Autodesk Inventor part; units mm, degrees
sketch "Esboço1" plane through (0, 0, 0) normal (0, 1, 0) x (-1, 0, 0)
  line L0 (-50, 50) -> (50, 50)
  line L1 (50, 50) -> (50, -50)
  line L2 (50, -50) -> (-50, -50)
  line L3 (-50, -50) -> (-50, 50)
  line L4 (-50, 50) -> (50, -50) construction
  line L5 (50, 50) -> (-50, -50) construction
  line L6 (-40, 40) -> (40, 40)
  line L7 (40, 40) -> (40, -40)
  line L8 (40, -40) -> (-40, -40)
  line L9 (-40, -40) -> (-40, 40)
  line L10 (-40, 40) -> (40, -40) construction
  line L11 (40, 40) -> (-40, -40) construction
  point P0 (0, 0)
  dimension "d0" = 100
  dimension "d1" = 10
extrude "Extrusão1" add sketch "Esboço1" along normal mid plane 740
equation "\"Raio_vergadura\" = Espessura"
equation "\"Largura_alívio_de_vergadura\" = Espessura"
equation "\"Profundidade_alívio_de_vergadura\" = 0.5 * Espessura"
equation "\"Tamanho_alívio_de_dobra\" = 4 * Espessura"
equation "\"Remanescente_mínimo\" = 2 * Espessura"
equation "\"Raiodetransição\" = Raio_vergadura"
equation "\"Tamanho_de_raio_de_Jacobi\" = Raio_vergadura"
equation "\"TamanhoFolga\" = Espessura"
properties part number "Perna para Exercício"
Build history of the part. All positions in model axes, mm. A direction names the side the tool comes from. Coordinates: 2 decimals unless noted, no trailing zeros. Order: outer loops, then holes, each group sorted by start corner. A loop starts at its lowest first (then second) coordinate and runs counter-clockwise, first axis right, second up. Notation, with made-up numbers: M 23.5,30.25 L 73.5,30.25 A27 ccw 73.5,63.25 Z; hole C -34.5,-39.75 d10. An arc over 180 degrees is marked long. One line per question, with ' | ' between items. Start each with the question number.
1. Cut at B-B (z = 12.5). Write the cut outline in (x, y), plus the area to 3 significant figures.
2. Flat gauge pin, fed straight in: P1, Ø2, axis at x = 5, z = 39.5, coming from the +Y side. Where does the tip first touch, or does it go through?
3. Wall check: line 1 along X through (y, z) = (162, -31). Give the ranges that are in metal, low to high. Write a range as [from, to].
4. Tool access for faces 5 (the face through (1, -5, 40)), 6 (the face through (-50, -5, 1)): list every direction of +Z, -Z, +X, -X, +Y, -Y with a clear straight run to the whole face (end or side of a thin tool).
5. Mould opens along Z. For faces 1 (the face through (1, -5, 50)), 2 (the face through (-40, -5, 1)), 3 (the face through (-1, -5, -50)), 4 (the face through (45, -370, 1)) say: +Z half, -Z half, draft (parallel to the pull), parting line (faces both ways), or undercut.
6. Cut at C-C (y = -161). Write the cut outline in (x, z).
7. Cut at A-A (x = 30). Write the cut outline in (y, z), plus the area to 3 significant figures.
The answers:
1) outline: M -50,-370 L -40,-370 L -40,370 L -50,370 Z; M 40,-370 L 50,-370 L 50,370 L 40,370 Z | area: 14,800 mm2
2) P1: stops at y = 370
3) line 1: x = [-50, -40], [40, 50]
4) face 5: +Y, -Y | face 6: +Z, -Z, -X, +Y, -Y
5) face 1: +Z half | face 2: undercut | face 3: -Z half | face 4: draft
6) outline: M -50,-50 L 50,-50 L 50,50 L -50,50 Z; hole M -40,-40 L 40,-40 L 40,40 L -40,40 Z
7) outline: M -370,-50 L 370,-50 L 370,-40 L -370,-40 Z; M -370,40 L 370,40 L 370,50 L -370,50 Z | area: 14,800 mm2
